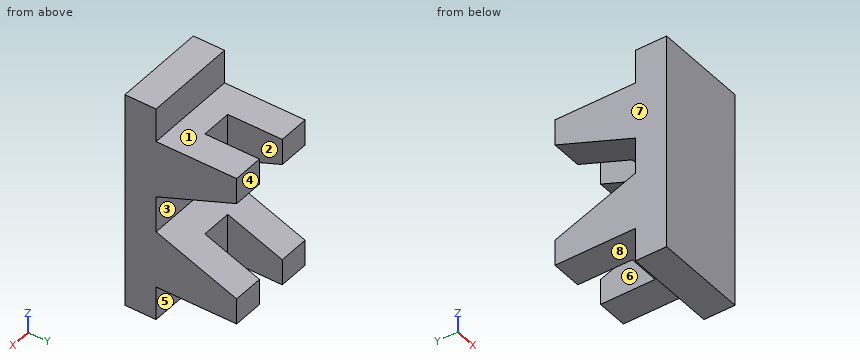
from build123d import *

# Parameters (mm, degrees)
SALIENTE_EXTRUIR1_DEPTH = 36
CROQUIS2_W              = 12
CROQUIS2_H              = 21
CORTAR_EXTRUIR1_DEPTH   = 91.47651629


with BuildPart() as part:
    # Croquis1 → Saliente-Extruir1 (new body)
    with BuildSketch(Plane(origin=(0, 0, 0), x_dir=(0, 0, -1), z_dir=(1, 0, 0))):
        Polygon((42, 0), (-42, 0), (-42, 12), (-29, 12), (-29, 43), (-19, 43), (-7, 12), (7, 12), (19, 43), (29, 43), (29, 12), (42, 12), align=None)
    extrude(amount=SALIENTE_EXTRUIR1_DEPTH)

    # Croquis2 → Cortar-Extruir1 (cut, through all)
    with BuildSketch(Plane.XY.offset(29)):
        with Locations((18, 32.5)):
            Rectangle(CROQUIS2_W, CROQUIS2_H)
    extrude(amount=-CORTAR_EXTRUIR1_DEPTH, mode=Mode.SUBTRACT)


solid = part.part
Verification items for the finished model (mm, model axes). Face numbers are marked on the shaded views. A direction names the side the tool comes from. Coordinates: 2 decimals unless noted, no trailing zeros. Write each loop counter-clockwise with the first axis right and the second up, starting at its lowest first coordinate (ties: lowest second). Pieces come first, ordered by that corner, then holes. Notation, with made-up numbers: M -11,80 L 0,80 A9 ccw 0,92 Z; hole C -27.75,-2.75 d7. An arc over 180 degrees is marked long. Use a Markdown table: item, result.
Q1. Draft check along X on the marked faces 6, 7 and 8. Enter one of: +X half, -X half, draft (parallel to the pull), parting line (faces both ways), or undercut.
Reply:
| item | result |
|---|---|
| face 6 | undercut |
| face 7 | -X half |
| face 8 | draft |
Q2. Sectioned sample at D-D, the plane x = 25.5. Record the boundary of the cut face in (y, z).
Reply:
| item | result |
|---|---|
| outline | M 0,-42 L 12,-42 L 12,-29 L 43,-29 L 43,-19 L 12,-7 L 12,7 L 43,19 L 43,29 L 12,29 L 12,42 L 0,42 Z |
Q3. Sectioned sample at B-B, the plane z = 26. Record the boundary of the cut face in (x, y).
Reply:
| item | result |
|---|---|
| outline | M 0,0 L 36,0 L 36,43 L 24,43 L 24,22 L 12,22 L 12,43 L 0,43 Z |
Q4. Set-up check for the marked faces 1, 2, 3, 4 and 5: record each of +Z, -Z, +X, -X, +Y, -Y from which the full face is reachable in a straight line by a thin tool's end or side.
Reply:
| item | result |
|---|---|
| face 1 | +Z, +X, -X, +Y |
| face 2 | +Z, -Z, +Y |
| face 3 | +X, -X, +Y |
| face 4 | +Z, -Z, +X, -X, +Y |
| face 5 | -Z, +X, -X, +Y |
Q5. Sectioned sample at A-A, the plane y = 35. Record the boundary of the cut face in (x, z), plus the area to 3 significant figures.
Reply:
| item | result |
|---|---|
| outline | M 0,-29 L 12,-29 L 12,-15.9 L 0,-15.9 Z; M 0,15.9 L 12,15.9 L 12,29 L 0,29 Z; M 24,-29 L 36,-29 L 36,-15.9 L 24,-15.9 Z; M 24,15.9 L 36,15.9 L 36,29 L 24,29 Z |
| area | 629 mm² |
Q6. Thickness scan on line 1 (X direction, y = 22.5, z = 18.5); line 2 (Y direction, x = 23, z = 38.5); line 3 (Z direction, x = 2, y = 19). Record the ranges inside material, lowest first.
Reply:
| item | result |
|---|---|
| line 1 | x = 0 to 12, 24 to 36 |
| line 2 | y = 0 to 12 |
| line 3 | z = -29 to -9.71, 9.71 to 29 |
Q7. Sectioned sample at C-C, the plane y = 18. Record the boundary of the cut face in (x, z).
Reply:
| item | result |
|---|---|
| outline | M 0,-29 L 36,-29 L 36,-9.32 L 0,-9.32 Z; M 0,9.32 L 36,9.32 L 36,29 L 0,29 Z |
Q8. Go/stop test with flat-tipped pins: P1, Ø14.5, axis at x = 24.5, z = 38.5, coming from the +Y side; P2, Ø1, axis at x = 11, z = 26.5, coming from the -Y side; P3, Ø6, axis at x = 16.5, z = 16.5, coming from the +Y side; P4, Ø8, axis at x = 8.5, y = 16.5, coming from the +Z side. Record where each tip stops, or that it passes through.
Reply:
| item | result |
|---|---|
| P1 | stops at y = 12 |
| P2 | stops at y = 0 |
| P3 | stops at y = 22 |
| P4 | stops at z = 29 |
